from build123d import *

# Parameters (mm, degrees)
F0_R     = 51.59375
F1_DEPTH = 9.525
F2_R     = 38.89375
F3_DEPTH = 22.225
F4_W     = 12.7
F4_H     = 2.54
F7_D     = 19.05


with BuildPart() as f1:
    # F0 (on Right) → F1 (new body, symmetric)
    with BuildSketch(Plane.YZ):
        Circle(F0_R)
    extrude(amount=F1_DEPTH, both=True)

    # F2 (on face) → F3 (join)
    with BuildSketch(Plane.YZ.offset(9.525)):
        Circle(F2_R)
    extrude(amount=F3_DEPTH)

    # F4 (on Front) → F5 (revolve, cut)
    with BuildSketch(Plane.XZ):
        with Locations((0, 51.59375)):
            Rectangle(F4_W, F4_H)
    revolve(axis=Axis((1.883045, 0, 0), (1, 0, 0)), mode=Mode.SUBTRACT)

    # F7 (through all)
    with Locations(Plane.YZ.offset(31.75)):
        with Locations((0, 0)):
            Hole(F7_D / 2)


solid = f1.part
Design review of the part built by this model. Coordinates are the model's own, in mm. A direction names the side the tool comes from. Give positions to 0.01 mm unless a question says otherwise; leave off trailing zeros. Loops run counter-clockwise (first coordinate to the right, second up) from the corner with the lowest first, then second, coordinate; pieces in that order, holes last. Notation, with made-up numbers: (0.25, 63) - (47.25, 63) arc R32 ccw to (47.25, 93) - close; hole circle Ø10 at (35, 82). An arc over 180 degrees is marked (long way). Use CSV: the item, a comma, the result in double quotes. Start each with the question number.
1. Insertion check: P1, Ø5, axis at x = 12.5, y = -35.5, coming from the -Z side; P2, Ø1, axis at x = 27, z = -36.5, coming from the +Y side; P3, Ø12, axis at x = 25, z = -31, coming from the -Y side. Each pin has a flat end and moves straight along its axis. Give the tip position at first contact, or say it passes through.
2. Add section D-D (y = 11). State the section outline as (x, z) points (3 decimals), plus the area to 3 significant figures.
3. Machinability: for faces 4 (the flat face through (6.35, 11.2, -49.4)), 5 (the flat face through (31.75, 8, -8)), 6 (the cylindrical face through (20.48, -30.86, -23.67)), which of the approach directions +Z, -Z, +X, -X, +Y, -Y give a long, thin tool a straight path to every point of the face, cutting with its end or side? Answer none if there is none.
4. Wall thickness on L1, parallel to Z at x = 9, y = 0 (3 decimals); L2, parallel to Z at x = 19.5, y = 0 (3 decimals); L3, parallel to X at y = -19.5, z = 47 (3 decimals): over which ranges is each line inside the solid? List them lowest first.
5. Add section A-A (y = 0). State the section outline as (x, z) points (3 decimals).
6. Draft analysis for pull direction X (two halves, no side actions). For faces 1 (the flat face through (-6.35, 11.2, -49.4)), 2 (the flat face through (9.525, 7.4, 38.5)), 3 (the cylindrical face through (-7.915, -40.943, -31.394)), state which applies: released by +X, released by -X, zero draft, split by the parting line, or undercut.
Results found:
1,P1,"stops at z = -20.58"
1,P2,"stops at y = 14.72"
1,P3,"stops at y = -29.79"
2,outline,"(-9.525, -50.407) - (-6.35, -50.407) - (-6.35, -49.107) - (6.35, -49.107) - (6.35, -50.407) - (9.525, -50.407) - (9.525, -37.306) - (31.75, -37.306) - (31.75, 37.306) - (9.525, 37.306) - (9.525, 50.407) - (6.35, 50.407) - (6.35, 49.107) - (-6.35, 49.107) - (-6.35, 50.407) - (-9.525, 50.407) - close"
2,area,"3,550 mm²"
3,face 4,"none"
3,face 5,"+Z, -Z, +X, +Y, -Y"
3,face 6,"+X"
4,L1,"z = -51.594 to -9.525, 9.525 to 51.594"
4,L2,"z = -38.894 to -9.525, 9.525 to 38.894"
4,L3,"x = -9.525 to -6.35, 6.35 to 9.525"
5,outline,"(-9.525, -51.594) - (-6.35, -51.594) - (-6.35, -50.324) - (6.35, -50.324) - (6.35, -51.594) - (9.525, -51.594) - (9.525, -38.894) - (31.75, -38.894) - (31.75, -9.525) - (-9.525, -9.525) - close; (-9.525, 9.525) - (31.75, 9.525) - (31.75, 38.894) - (9.525, 38.894) - (9.525, 51.594) - (6.35, 51.594) - (6.35, 50.324) - (-6.35, 50.324) - (-6.35, 51.594) - (-9.525, 51.594) - close"
6,face 1,"undercut"
6,face 2,"released by +X"
6,face 3,"zero draft"
